Could you check a few things on this drawing? It's one solid part, dimensions in mm from its lowest x, y, z. A direction names the side the tool comes from. Give positions to 0.01 mm unless a question says otherwise; leave off trailing zeros. Loops run counter-clockwise (first coordinate to the right, second up) from the corner with the lowest first, then second, coordinate; pieces in that order, holes last.
1. Imagine slicing it at A-A (z = 11). List the corners of the cut face in (x, y) for me, plus the area to 3 significant figures.
2. For the marked faces 1, 2 and 3, which set-ups out of +Z, -Z, +X, -X, +Y, -Y let a thin tool reach every point of the face, with its end or its side?
3. Imagine slicing it at B-B (y = 32). List the corners of the cut face in (x, z) for me, plus the area to 3 significant figures.
4. Imagine slicing it at C-C (x = 24). List the corners of the cut face in (y, z) for me.
5. For P1, Ø2, axis at y = 28.5, z = 5, coming from the +X side; P2, Ø1, axis at x = 10.5, y = 10.5, coming from the -Z side; P3, Ø10, axis at x = 17, z = 21, coming from the -Y side; P4, Ø2, axis at x = 27, y = 30, coming from the +Z side, each with a flat end and sliding along its axis, tell me the tip position at first contact or that it passes through.
6. I need wall thicknesses on line 1 along X through (y, z) = (22.5, 6.25); line 2 along Y through (x, z) = (34.5, 9.75); line 3 along Y through (x, z) = (9, 18.25). Which ranges of each line are inside material? Lowest first, please.
7. Imagine slicing it at D-D (x = 5). List the corners of the cut face in (y, z) for me.
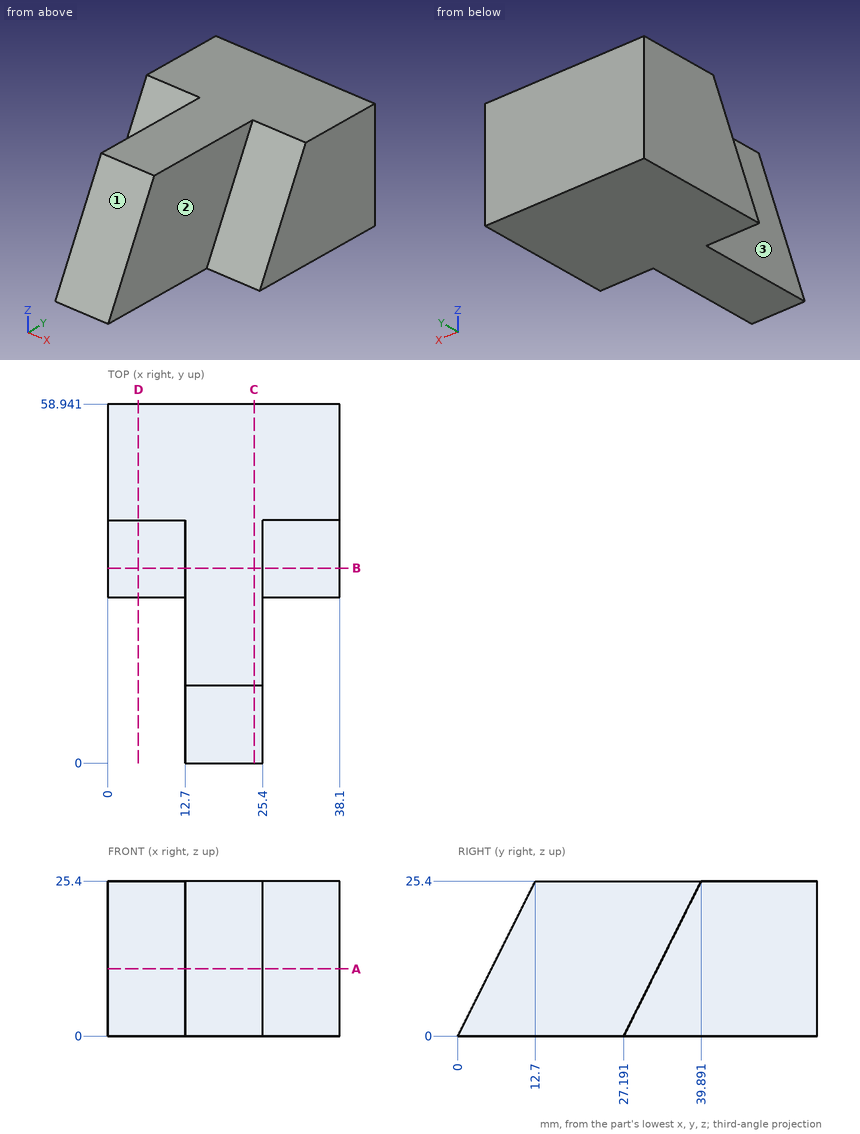
Derived:
1. outline: (0, 32.69) - (12.7, 32.69) - (12.7, 5.5) - (25.4, 5.5) - (25.4, 32.69) - (38.1, 32.69) - (38.1, 58.94) - (0, 58.94) - close
1. area: 1,350 mm2
2. face 1: +Z, +X, -X, -Y
2. face 2: +Z, +X, -Y
2. face 3: +Z, -X, -Y
3. outline: (0, 0) - (38.1, 0) - (38.1, 9.62) - (25.4, 9.62) - (25.4, 25.4) - (12.7, 25.4) - (12.7, 9.62) - (0, 9.62) - close
3. area: 567 mm2
4. outline: (0, 0) - (58.94, 0) - (58.94, 25.4) - (12.7, 25.4) - close
5. P1: stops at x = 25.4
5. P2: passes through
5. P3: stops at y = 8
5. P4: stops at z = 7.62
6. line 1: x = 12.7 to 25.4
6. line 2: y = 32.07 to 58.94
6. line 3: y = 36.32 to 58.94
7. outline: (27.19, 0) - (58.94, 0) - (58.94, 25.4) - (39.89, 25.4) - close
